Study the drawing (mm; zero at the part's minimum x, y, z) and answer. Round coordinates to 2 decimals unless told otherwise and drop trailing zeros. Loops run counter-clockwise (first coordinate to the right, second up) from the corner with the lowest first, then second, coordinate; pieces in that order, holes last. Notation, with made-up numbers: (-33.5, 5.5) -> (-6.5, 5.5) arc R30 ccw to (-6.5, 35.5) -> close; hole circle Ø9 at (85, 26.5). An arc over 180 degrees is marked (long way). Answer in a Markdown table with one row per item. Add a question column.
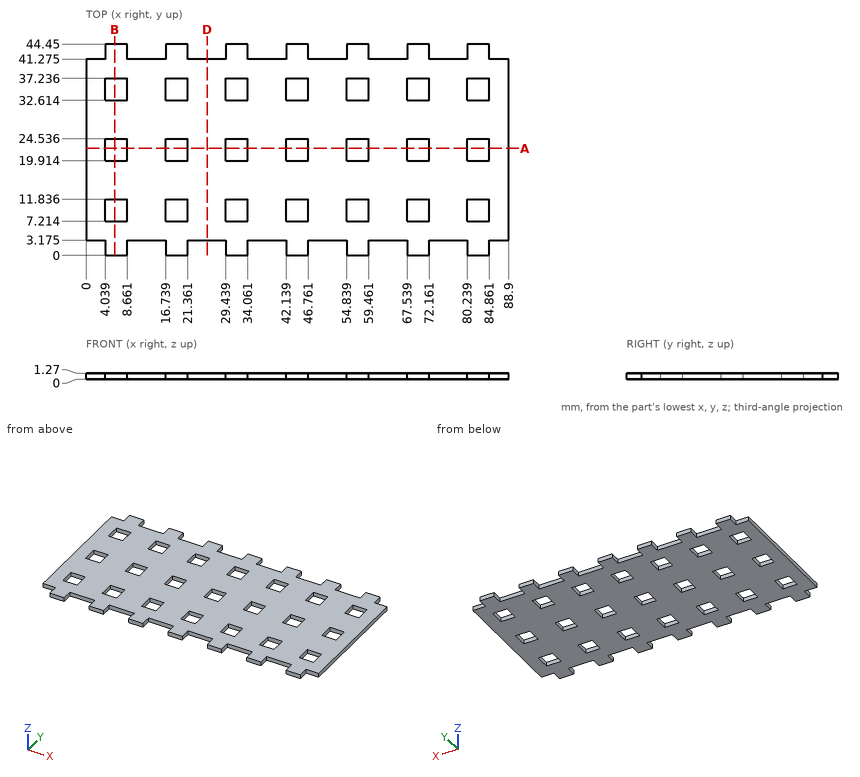
Item 1: Section D-D, the plane x = 25.5 is taken. Write down the section's boundary in (y, z) (1 decimal).
Item 2: Consider L1, parallel to Y at x = 21, z = 0.7; L2, parallel to Y at x = 38, z = 0.8 (1 decimal). Determine where each line is inside the solid, lowest interval first. Write a range as from..to.
Item 3: Section B-B, the plane x = 6 is taken. Write down the section's boundary in (y, z).
Item 4: Section A-A, the plane y = 22.5 is taken. Give the number of separate pieces and of enclosed holes in the cut face.
Item 5: A flat-ended cylindrical pin translates along its axis: P1, Ø0.6, axis at y = 43.5, z = 0.5, coming from the -X side. Find the tip coordinate at first contact, or state that the pin passes through.
Here are the results:
| question | item | result |
|---|---|---|
| 1 | outline | (3.2, 0) -> (41.3, 0) -> (41.3, 1.3) -> (3.2, 1.3) -> close |
| 2 | L1 | y = 0..7.21, 11.84..19.91, 24.54..32.61, 37.24..44.45 |
| 2 | L2 | y = 3.2..41.3 |
| 3 | outline | (0, 0) -> (7.21, 0) -> (7.21, 1.27) -> (0, 1.27) -> close; (11.84, 0) -> (19.91, 0) -> (19.91, 1.27) -> (11.84, 1.27) -> close; (24.54, 0) -> (32.61, 0) -> (32.61, 1.27) -> (24.54, 1.27) -> close; (37.24, 0) -> (44.45, 0) -> (44.45, 1.27) -> (37.24, 1.27) -> close |
| 4 | separate pieces | 8 |
| 4 | enclosed holes | 0 |
| 5 | P1 | stops at x = 4.04 |
